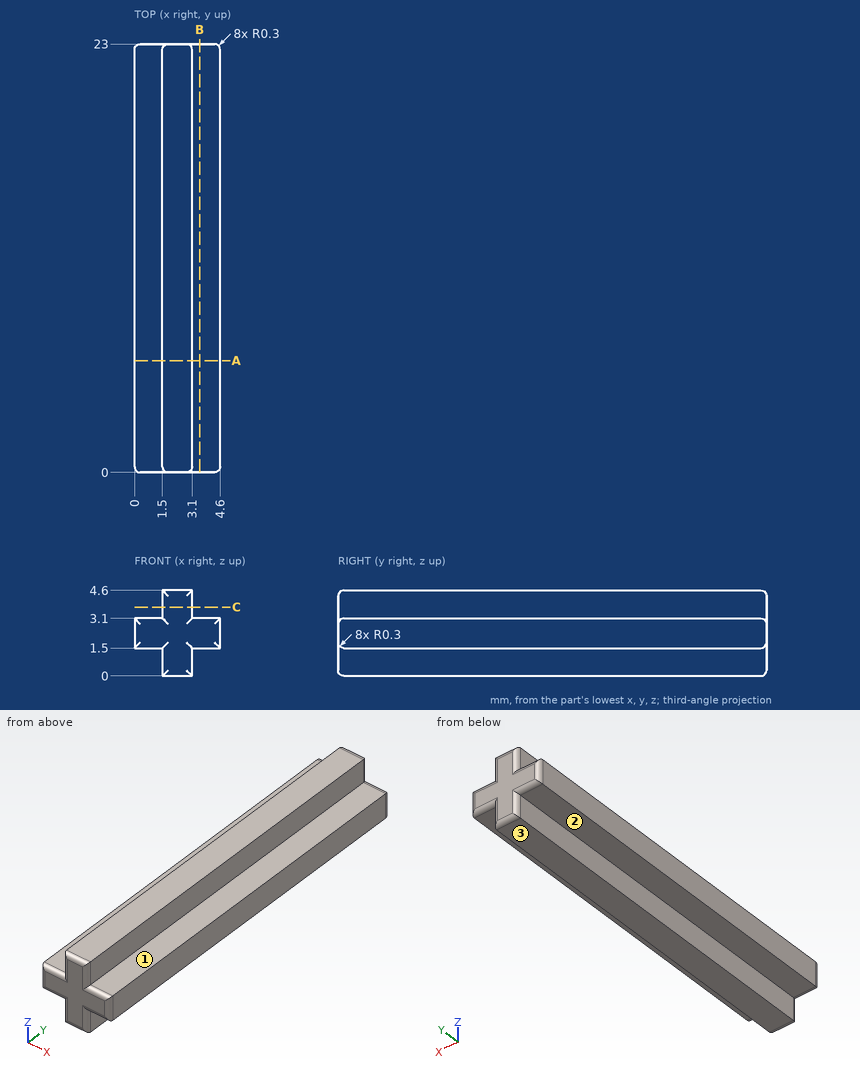
Study the drawing (mm; zero at the part's minimum x, y, z) and answer. A direction names the side the tool comes from. Coordinates: 2 decimals unless noted, no trailing zeros. Order: outer loops, then holes, each group sorted by start corner. A loop starts at its lowest first (then second) coordinate and runs counter-clockwise, first axis right, second up. Notation, with made-up numbers: M -6.75,-6.75 L 34.25,-6.75 A13 ccw 34.25,10.25 Z; hole C -39,76.25 d2. An arc over 180 degrees is marked long. Use CSV: the item, a comma, the result in double quotes.
Q1. Straight lines are drawn through the part: L1, parallel to X at y = 1.75, z = 4.45; L2, parallel to Y at x = 4.1, z = 2.85. For each, find the intervals that lie inside material, in ascending order.
Here are the results:
L1,"1.5 to 3.1"
L2,"0 to 23"
Q2. A tool of negligible diameter and unlimited length cuts with its end or side. For the marked faces 1, 2 and 3, from which of +Z, -Z, +X, -X, +Y, -Y can it reach the whole face along a straight path? Write none if from no direction.
Here are the results:
face 1,"+Z, +X, +Y, -Y"
face 2,"-Z, -X, +Y, -Y"
face 3,"-Z, +X, -X, +Y, -Y"
Q3. Section A-A (y = 6) is taken. Determine the outline of the cut face in (x, z).
Here are the results:
outline,"M 0,1.5 L 1.5,1.5 L 1.5,0 L 3.1,0 L 3.1,1.5 L 4.6,1.5 L 4.6,3.1 L 3.1,3.1 L 3.1,4.6 L 1.5,4.6 L 1.5,3.1 L 0,3.1 Z"
Q4. Section B-B (x = 3.5) is taken. Determine the outline of the cut face in (y, z).
Here are the results:
outline,"M 0,1.8 A0.3 ccw 0.3,1.5 L 22.7,1.5 A0.3 ccw 23,1.8 L 23,2.8 A0.3 ccw 22.7,3.1 L 0.3,3.1 A0.3 ccw 0,2.8 Z"
Q5. Section C-C (z = 3.7) is taken. Determine the outline of the cut face in (x, y), then the cut area to 3 significant figures.
Here are the results:
outline,"M 1.5,0.3 A0.3 ccw 1.8,0 L 2.8,0 A0.3 ccw 3.1,0.3 L 3.1,22.7 A0.3 ccw 2.8,23 L 1.8,23 A0.3 ccw 1.5,22.7 Z"
area,"36.7 mm2"
Q6. Given pin 1 Ø1.2 at (x, y) = (4, 12.5) entering from -Z; pin 2 Ø0.7 at (x, y) = (0.5, 9) entering from +Z; pin 3 Ø0.7 at (y, z) = (8.5, 0.5) entering from -X, each flat-ended and moving along its own axis, determine where each tip first touches the part or whether it passes through.
Here are the results:
pin 1,"z = 1.5"
pin 2,"z = 3.1"
pin 3,"x = 1.5"
